```python
from build123d import *

# Parameters (mm, degrees)
BOSS_EXTRUDE1_DEPTH = 13.97
SKETCH3_W           = 1.016
SKETCH3_H           = 3.81
CUT_EXTRUDE1_DEPTH  = 14.97
CUT_EXTRUDE2_DEPTH  = 2.27


with BuildPart() as part:
    # Sketch1 → Boss-Extrude1 (new body)
    with BuildSketch(Plane.XY):
        Polygon((0, 0), (0, 20.32), (-12.7, 20.32), (-12.7, 0), (-14.605, 0), (-14.605, 19.05), (-14.605, 25.4), (1.905, 25.4), (1.905, 19.05), (1.905, 0), align=None)
    extrude(amount=-BOSS_EXTRUDE1_DEPTH)

    # Sketch3 → Cut-Extrude1 (cut, through all)
    with BuildSketch(Plane.XY):
        with Locations((-0.508, 22.225)):
            Rectangle(SKETCH3_W, SKETCH3_H)
    extrude(amount=-CUT_EXTRUDE1_DEPTH, mode=Mode.SUBTRACT)

    # Sketch4 → Cut-Extrude2 (cut, through all)
    with BuildSketch(Plane.XZ.offset(-24.13)):
        Polygon((-1.016, -6.985), (-1.016, -3.175), (0, -3.175), (0, -10.795), (-1.016, -10.795), align=None)
    extrude(amount=-CUT_EXTRUDE2_DEPTH, mode=Mode.SUBTRACT)


solid = part.part
```
Geometry: final body of the model. Coordinates: model frame, mm. A direction names the side the tool comes from. Round coordinates to 2 decimals unless told otherwise and drop trailing zeros. Order: outer loops, then holes, each group sorted by start corner. A loop starts at its lowest first (then second) coordinate and runs counter-clockwise, first axis right, second up. Notation, with made-up numbers: (24, 23) -> (39, 23) arc R19 ccw to (39, 55) -> close; hole circle Ø4 at (66, 29.5). An arc over 180 degrees is marked (long way). Use one line per item in the form item = value. Start each with the question number.
1. Pin query (flat end, axial travel): pin 1 Ø0.5 at (x, z) = (-0.5, -12.5) entering from -Y; pin 2 Ø3 at (x, z) = (-7, -1.5) entering from -Y. Return the tip coordinate at first contact, or that it passes through.
2. Reachability of faces 4 (the face through (-12.7, 10, -7)), 5 (the face through (-0.5, 24.8, -3.175)), 6 (the face through (-6, 21, 0)), 7 (the face through (-14, 0, -7)), 8 (the face through (-1.016, 23, -7)) from +Z, -Z, +X, -X, +Y, -Y: full face, straight path, thin tool, end or side. Return the list, or none.
3. Line query: probe 1 along X at (y, z) = (15.75, -3) (3 decimals); probe 2 along X at (y, z) = (23.5, -3.75) (3 decimals); probe 3 along Y at (x, z) = (-3, -9.5). Output: solid intervals per line, ascending.
4. Cut plane B-B (z = -9). Return the cut outline in (x, y) (3 decimals).
5. Cut plane D-D (z = -1.75). Return the cut outline in (x, y) (3 decimals).
6. Cut plane A-A (y = 6.5). Return the cut outline in (x, z) (3 decimals).
7. Cut plane C-C (y = 22). Return the cut outline in (x, z) (3 decimals).
8. Draft query along X for faces 1 (the face through (-7, 20.32, -7)), 2 (the face through (1, 0, -7)), 3 (the face through (-14.605, 13, -7)). Return one class per face: pulls with the +X half, pulls with the -X half, needs draft (parallel to the pull), parting line crosses it, or undercut.
Solution:
q1.pin_1 = 24.13
q1.pin_2 = 20.32
q2.face_4 = +Z, -Z, -Y
q2.face_5 = +Y, -Y
q2.face_6 = +Z, +X, -X, +Y, -Y
q2.face_7 = +Z, -Z, +X, -X, -Y
q2.face_8 = -Y
q3.probe_1 = -14.605 to -12.7, 0 to 1.905
q3.probe_2 = -14.605 to -1.016, 0 to 1.905
q3.probe_3 = 20.32 to 25.4
q4.outline = (-14.605, 0) -> (-12.7, 0) -> (-12.7, 20.32) -> (-1.016, 20.32) -> (-1.016, 25.4) -> (-14.605, 25.4) -> close; (0, 0) -> (1.905, 0) -> (1.905, 25.4) -> (0, 25.4) -> close
q5.outline = (-14.605, 0) -> (-12.7, 0) -> (-12.7, 20.32) -> (-1.016, 20.32) -> (-1.016, 24.13) -> (0, 24.13) -> (0, 0) -> (1.905, 0) -> (1.905, 25.4) -> (-14.605, 25.4) -> close
q6.outline = (-14.605, -13.97) -> (-12.7, -13.97) -> (-12.7, 0) -> (-14.605, 0) -> close; (0, -13.97) -> (1.905, -13.97) -> (1.905, 0) -> (0, 0) -> close
q7.outline = (-14.605, -13.97) -> (-1.016, -13.97) -> (-1.016, 0) -> (-14.605, 0) -> close; (0, -13.97) -> (1.905, -13.97) -> (1.905, 0) -> (0, 0) -> close
q8.face_1 = undercut
q8.face_2 = needs draft
q8.face_3 = pulls with the -X half
